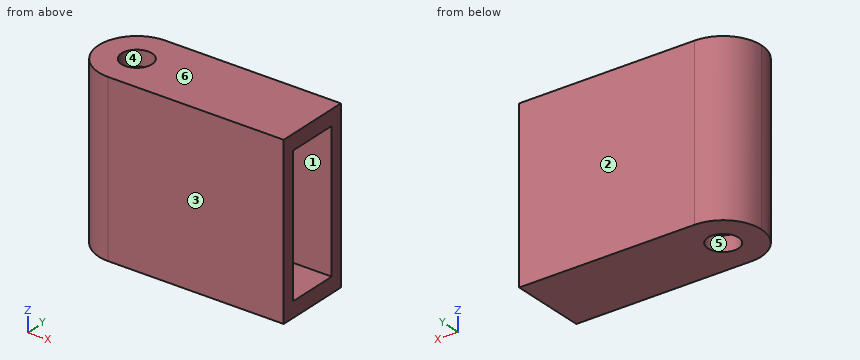
Autodesk Inventor part; units mm, degrees
ref_plane "YZ Plane" through (0, 0, 0) normal (1, 0, 0) x (0, 1, 0)
ref_plane "XZ Plane" through (0, 0, 0) normal (0, 1, 0) x (-1, 0, 0)
ref_plane "XY Plane" through (0, 0, 0) normal (0, 0, 1) x (1, 0, 0)
sketch "Sketch1" plane through (0, 0, 0) normal (0, 0, 1) x (1, 0, 0)
  line L0 (-40, 12.5) -> (40, 12.5)
  line L1 (40, 12.5) -> (40, -12.5)
  line L2 (40, -12.5) -> (-40, -12.5)
  line L3 (-40, -12.5) -> (-40, 12.5)
  line L4 (-40, 12.5) -> (40, -12.5) construction
  line L5 (40, 12.5) -> (-40, -12.5) construction
  point P0 (0, 0)
  dimension "d0" = 80
  dimension "d1" = 25
extrude "Extrusion1" add sketch "Sketch1" along normal blind 55
sketch "Sketch2" plane through (0, 0, 55) normal (0, 0, 1) x (1, 0, 0)
  circle A0 centre (-27.5, 0) radius 5
  line L0 (-40, 12.5) -> (-40, -12.5)
  point P0 (0, 0)
  dimension "d4" = 10
  dimension "d5" = 12.5
extrude "Extrusion2" cut sketch "Sketch2" against normal through all
sketch "Sketch3" plane through (40, -12.5, 0) normal (1, 0, 0) x (0, 0, -1)
  line L0 (-50, 4) -> (-5, 4)
  line L1 (-5, 4) -> (-5, 21)
  line L2 (-5, 21) -> (-50, 21)
  line L3 (-50, 21) -> (-50, 4)
  line L4 (-50, 4) -> (-5, 21) construction
  line L5 (-5, 4) -> (-50, 21) construction
  line L6 (-55, 0) -> (-55, 25)
  line L7 (0, 25) -> (-55, 25)
  point P0 (0, 12.5)
  point P1 (-27.5, 12.5)
  dimension "d8" = 45
  dimension "d9" = 17
  dimension "d10" = 27.5
  dimension "d11" = 12.5
extrude "Extrusion3" cut sketch "Sketch3" against normal blind 73.25
full round fillet "Full Round Fillet1" first side at (15.5833, 8.5, 20) centre faces at (-33.25, -2.8333, 20) second side at (15.5833, -8.5, 35)
fillet "Fillet1" radius 12.5 2 edges at (-40, 12.5, 27.5) (-40, -12.5, 27.5)
sketch "Sketch4" plane through (40, -12.5, 0) normal (1, 0, 0) x (0, 0, -1)
  line L0 (-55, 0) -> (-55, 25)
  line L1 (0, 0) -> (-55, 0)
  line L2 (-55, 25) -> (0, 25)
  line L3 (0, 25) -> (0, 0)
  line L4 (0, 0) -> (-55, 0)
  line L5 (-55, 0) -> (-55, 25)
  point P0 (0, 12.5)
extrude "Extrusion4" cut sketch "Sketch4" against normal blind 10
properties part number "2nd arm"
CAD build for the part. Positions are in the model's coordinates, mm. Face numbers are marked on the shaded views. A direction names the side the tool comes from. Round coordinates to 2 decimals unless told otherwise and drop trailing zeros. Write each loop counter-clockwise with the first axis right and the second up, starting at its lowest first coordinate (ties: lowest second). Pieces come first, ordered by that corner, then holes. Notation, with made-up numbers: M 67.5,8 L 72.5,8 A34 ccw 72.5,41 Z; hole C 70.5,22 d1. An arc over 180 degrees is marked long. Put each result on its own line as item: value. Start each with the question number.
1) Saw through at B-B, the plane x = 25. Write the cut outline in (y, z), and give its area (3 significant figures).
2) Pull direction Y, two halves, no side cores. Call the marked faces 3, 4, 5 and 6: pulls with the +Y half, pulls with the -Y half, needs draft (parallel to the pull), parting line crosses it, or undercut.
3) Saw through at C-C, the plane y = -3.75. Write the cut outline in (x, z), and give its area (3 significant figures).
4) Drill centre lines: probe 1 along Y at (x, z) = (-27.5, 52.9); probe 2 along Z at (x, y) = (2.5, 6.5); probe 3 along Y at (x, z) = (18, 44). Where is each one in solid material? Low to high. Write a range as [from, to].
5) Pin check, flat tips, straight feed: pin 1 Ø10 at (y, z) = (9.5, 33.5) entering from -X; pin 2 Ø3 at (y, z) = (-6, 42.5) entering from +X. Stop position of each tip, or through.
6) 3-axis set-ups, long thin cutter, end or side, ignore diameter. For the marked faces 1 and 2: which of +Z, -Z, +X, -X, +Y, -Y reach the whole face in a straight line?
Resolved:
1. outline: M -12.5,0 L 12.5,0 L 12.5,55 L -12.5,55 Z; hole M -8.5,5 L 8.5,5 L 8.5,50 L -8.5,50 Z
1. area: 610 mm²
2. face 3: pulls with the -Y half
2. face 4: undercut
2. face 5: undercut
2. face 6: needs draft
3. outline: M -39.42,0 L -30.81,0 L -30.81,5 L -32.38,5 L -32.38,50 L -30.81,50 L -30.81,55 L -39.42,55 Z; M -24.19,0 L 30,0 L 30,5 L -24.19,5 Z; M -24.19,50 L 30,50 L 30,55 L -24.19,55 Z
3. area: 945 mm²
4. probe 1: [-12.5, -5], [5, 12.5]
4. probe 2: [0, 5], [50, 55]
4. probe 3: [-12.5, -8.5], [8.5, 12.5]
5. pin 1: x = -39.16
5. pin 2: x = -28.75
6. face 1: +X
6. face 2: +Z, -Z, +X, -X, +Y
